```python
from build123d import *

# Parameters (mm, degrees)
SKETCH1_R               = 20
BOSS_EXTRUDE1_DEPTH     = 200
CUT_EXTRUDE1_DEPTH      = 202.990098767
CUT_EXTRUDE1_DEPTH_BACK = 200
SKETCH2_R               = 10
SKETCH5_R               = 5
BOSS_EXTRUDE4_DEPTH     = 10


with BuildPart() as part:
    # Sketch1 → Boss-Extrude1 (new body)
    with BuildSketch(Plane(origin=(0, 0, 0), x_dir=(1, 0, 0), z_dir=(0, 1, 0))):
        with Locations(Location((0, 0, 0), (0, 0, 270))):
            Circle(SKETCH1_R)
    extrude(amount=BOSS_EXTRUDE1_DEPTH)

    # Sketch2 → Cut-Extrude1 (cut, two sides: drawn at the far end of the back side and taken through both)
    with BuildSketch(Plane.XY.offset(-CUT_EXTRUDE1_DEPTH_BACK)):
        with Locations(Location((0, 100, 0), (0, 0, 90))):
            Circle(SKETCH2_R)
    extrude(amount=CUT_EXTRUDE1_DEPTH + CUT_EXTRUDE1_DEPTH_BACK, mode=Mode.SUBTRACT)

    # Sketch5 → Boss-Extrude4 (add)
    with BuildSketch(Plane(origin=(0, 200, 0), x_dir=(1, 0, 0), z_dir=(0, 1, 0))):
        with Locations(Location((0, 0, 0), (0, 0, 270))):
            Circle(SKETCH5_R)
    extrude(amount=BOSS_EXTRUDE4_DEPTH)


solid = part.part
```
The listing builds one solid part. Answer for the finished solid, in the listing's coordinates (mm). A direction names the side the tool comes from. Coordinates: 2 decimals unless noted, no trailing zeros. Write each loop counter-clockwise with the first axis right and the second up, starting at its lowest first coordinate (ties: lowest second). Pieces come first, ordered by that corner, then holes. Notation, with made-up numbers: M 11,35.5 L 54,35.5 A18 cw 54,66.5 Z; hole C -14.75,48 d7. An arc over 180 degrees is marked long. Use a Markdown table: item, result. Add a question column.
1. Section D-D (x = -12) is taken. Give the vertices of the cut face in (y, z), plus the area to 3 significant figures.
2. Straight lines are drawn through the part: line 1 along Y through (x, z) = (0, -1.5); line 2 along Y through (x, z) = (0, 10); line 3 along Y through (x, z) = (-13, 9.5). For each, find the intervals that lie inside material, in ascending order. Write a range as [from, to].
3. Section A-A (x = 0) is taken. Give the vertices of the cut face in (y, z).
4. Which of the six approach directions +Z, -Z, +X, -X, +Y, -Y give full straight-line access (tool end or side, diameter ignored) to faces 1 (the flat face through (-4, 200, 4)), 2 (the cylindrical face through (-12, 99, -16))?
5. Section B-B (z = 0) is taken. Give the vertices of the cut face in (x, y), plus the area to 3 significant figures.
6. Section C-C (y = 22) is taken. Give the vertices of the cut face in (x, z), plus the area to 3 significant figures.
7. For a pull along X with two mould halves and no side action, classify faces 3 (the cylindrical face through (-8.43, 105.38, -0.28)), 4 (the cylindrical face through (-4.88, 204.93, -1.08)), 5 (the flat face through (0, 0, 0)) as +X half, -X half, draft (parallel to the pull), parting line (faces both ways), or undercut.
8. Given P1, Ø1, axis at y = 76.5, z = -7, coming from the +X side; P2, Ø3, axis at x = 15, y = 156.5, coming from the -Z side; P3, Ø4, axis at x = -13.5, y = 105, coming from the -Z side, each flat-ended and moving along its own axis, determine where each tip first touches the part or whether it passes through.
Data:
| question | item | result |
|---|---|---|
| 1 | outline | M 0,-16 L 200,-16 L 200,16 L 0,16 Z |
| 1 | area | 6,400 mm2 |
| 2 | line 1 | y = [0, 90], [110, 210] |
| 2 | line 2 | y = [0, 90], [110, 200] |
| 2 | line 3 | y = [0, 200] |
| 3 | outline | M 0,-20 L 90,-20 L 90,20 L 0,20 Z; M 110,-20 L 200,-20 L 200,-5 L 210,-5 L 210,5 L 200,5 L 200,20 L 110,20 Z |
| 4 | face 1 | +Y |
| 4 | face 2 | +Y, -Y |
| 5 | outline | M -20,0 L 20,0 L 20,200 L 5,200 L 5,210 L -5,210 L -5,200 L -20,200 Z; hole C 0,100 d20 |
| 5 | area | 7,790 mm2 |
| 6 | outline | C 0,0 d40 |
| 6 | area | 1,260 mm2 |
| 7 | face 3 | undercut |
| 7 | face 4 | parting line |
| 7 | face 5 | draft |
| 8 | P1 | stops at x = 18.91 |
| 8 | P2 | stops at z = -14.76 |
| 8 | P3 | stops at z = -16.36 |
